Verification items for the finished model (mm, model axes). Face numbers are marked on the shaded views. A direction names the side the tool comes from. Give positions to 0.01 mm unless a question says otherwise; leave off trailing zeros. Write each loop counter-clockwise with the first axis right and the second up, starting at its lowest first coordinate (ties: lowest second). Pieces come first, ordered by that corner, then holes. Notation, with made-up numbers: (27, -16) -> (82, -16) arc R28 cw to (82, 21) -> close; hole circle Ø2 at (5.5, -3.75). An arc over 180 degrees is marked (long way). Answer as CSV lines item,"result".
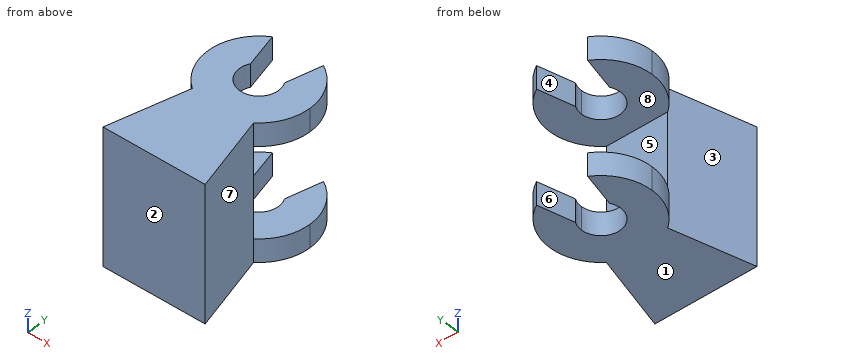
```python
from build123d import *

# Parameters (mm, degrees)
F1_DEPTH = 20
F2_DEPTH = 16.625
F3_DEPTH = 3.375


with BuildPart() as f1:
    # F0 (on Top) → F1 (new body)
    with BuildSketch(Plane.XY):
        with BuildLine():
            ThreePointArc((-11.25185, 21.143954), (-13.995725, 18.398907), (-15, 14.649832))
            ThreePointArc((-15, 14.649832), (-14.208204, 11.29573), (-12, 8.649832))
            Line((-12, 8.649832), (-3, 8.649832))
            ThreePointArc((-3, 8.649832), (-0.791796, 11.29573), (0, 14.649832))
            ThreePointArc((0, 14.649832), (-1.004275, 18.398907), (-3.74815, 21.143954))
            Line((-3.74815, 21.143954), (-5, 16.069559))
            ThreePointArc((-5, 16.069559), (-4.720331, 15.384041), (-4.625, 14.649832))
            ThreePointArc((-4.625, 14.649832), (-8.234209, 11.870163), (-10, 16.069559))
            Line((-10, 16.069559), (-11.25185, 21.143954))
        make_face()
        with BuildLine():
            Line((-12, 8.649832), (-15, -2.850168))
            Line((-15, -2.850168), (0, -2.850168))
            Line((0, -2.850168), (-3, 8.649832))
            ThreePointArc((-3, 8.649832), (-7.5, 7.149832), (-12, 8.649832))
        make_face()
        with BuildLine():
            Line((-3, 8.649832), (-12, 8.649832))
            ThreePointArc((-12, 8.649832), (-7.5, 7.149832), (-3, 8.649832))
        make_face()
    extrude(amount=F1_DEPTH)

    # F0 (on Top) → F2 (cut)
    with BuildSketch(Plane.XY):
        with BuildLine():
            ThreePointArc((-11.25185, 21.143954), (-13.995725, 18.398907), (-15, 14.649832))
            ThreePointArc((-15, 14.649832), (-14.208204, 11.29573), (-12, 8.649832))
            Line((-12, 8.649832), (-3, 8.649832))
            ThreePointArc((-3, 8.649832), (-0.791796, 11.29573), (0, 14.649832))
            ThreePointArc((0, 14.649832), (-1.004275, 18.398907), (-3.74815, 21.143954))
            Line((-3.74815, 21.143954), (-5, 16.069559))
            ThreePointArc((-5, 16.069559), (-4.720331, 15.384041), (-4.625, 14.649832))
            ThreePointArc((-4.625, 14.649832), (-8.234209, 11.870163), (-10, 16.069559))
            Line((-10, 16.069559), (-11.25185, 21.143954))
        make_face()
    extrude(amount=F2_DEPTH, mode=Mode.SUBTRACT)

    # F0 (on Top) → F3 (join)
    with BuildSketch(Plane.XY):
        with BuildLine():
            ThreePointArc((-11.25185, 21.143954), (-13.995725, 18.398907), (-15, 14.649832))
            ThreePointArc((-15, 14.649832), (-14.208204, 11.29573), (-12, 8.649832))
            Line((-12, 8.649832), (-3, 8.649832))
            ThreePointArc((-3, 8.649832), (-0.791796, 11.29573), (0, 14.649832))
            ThreePointArc((0, 14.649832), (-1.004275, 18.398907), (-3.74815, 21.143954))
            Line((-3.74815, 21.143954), (-5, 16.069559))
            ThreePointArc((-5, 16.069559), (-4.720331, 15.384041), (-4.625, 14.649832))
            ThreePointArc((-4.625, 14.649832), (-8.234209, 11.870163), (-10, 16.069559))
            Line((-10, 16.069559), (-11.25185, 21.143954))
        make_face()
    extrude(amount=F3_DEPTH)


solid = f1.part
```
1) Draft check along Y on the marked faces 6, 7 and 8. Enter one of: +Y half, -Y half, draft (parallel to the pull), parting line (faces both ways), or undercut.
Reported:
face 6,"+Y half"
face 7,"undercut"
face 8,"draft"
2) Section check D-D (z = 2). Record the boundary of the cut face in (x, y) (3 decimals), and give its area (3 significant figures).
Reported:
outline,"(-15, -2.85) -> (0, -2.85) -> (-3, 8.65) arc R7.5 ccw to (0, 14.65) arc R7.5 ccw to (-3.748, 21.144) -> (-5, 16.07) arc R2.875 cw to (-4.625, 14.65) arc R2.875 cw (long way) to (-10, 16.07) -> (-11.252, 21.144) arc R7.5 ccw to (-15, 14.65) arc R7.5 ccw to (-12, 8.65) -> close"
area,"248 mm²"
3) Scan lines: line 1 along Z through (x, y) = (-3, 18.25) (3 decimals); line 2 along Y through (x, z) = (-9.5, 9.75); line 3 along Y through (x, z) = (-7.5, 2.5). Record each from-to range of solid material in increasing order.
Reported:
line 1,"0 to 3.375, 16.625 to 20"
line 2,"-2.85 to 8.65"
line 3,"-2.85 to 11.77"
4) Depth check by flat-ended pin: pin 1 (4 mm diameter, centred on y = 8.5, z = 8.5, fed in from +X); pin 2 (1 mm diameter, centred on y = 6, z = 3.5, fed in from +X); pin 3 (4.5 mm diameter, centred on x = -9.5, z = 9, fed in from +Y). Enter the tip coordinate at first touch or a pass-through.
Reported:
pin 1,"x = -2.44"
pin 2,"x = -2.18"
pin 3,"y = 8.65"
5) Tool access check on the marked faces 1, 2, 3, 4 and 5. Record the directions out of +Z, -Z, +X, -X, +Y, -Y that give a thin tool (end or side, any length) a straight path to the whole face; none if there is none.
Reported:
face 1,"-Z, +X, -X, +Y, -Y"
face 2,"+Z, -Z, +X, -X, -Y"
face 3,"+Z, -Z, -X"
face 4,"+Z, -Z, +Y"
face 5,"+X, -X, +Y"
6) Section check C-C (y = 13). Record the boundary of the cut face in (x, z) (1 decimal).
Reported:
outline,"(-14.8, 0) -> (-9.9, 0) -> (-9.9, 3.4) -> (-14.8, 3.4) -> close; (-14.8, 16.6) -> (-9.9, 16.6) -> (-9.9, 20) -> (-14.8, 20) -> close; (-5.1, 0) -> (-0.2, 0) -> (-0.2, 3.4) -> (-5.1, 3.4) -> close; (-5.1, 16.6) -> (-0.2, 16.6) -> (-0.2, 20) -> (-5.1, 20) -> close"
7) Section check A-A (y = 10). Record the boundary of the cut face in (x, z) (3 decimals), and give its area (3 significant figures).
Reported:
outline,"(-13.385, 0) -> (-1.615, 0) -> (-1.615, 3.375) -> (-13.385, 3.375) -> close; (-13.385, 16.625) -> (-1.615, 16.625) -> (-1.615, 20) -> (-13.385, 20) -> close"
area,"79.4 mm²"
8) Section check B-B (x = -2.5). Record the boundary of the cut face in (y, z) (3 decimals), and give its area (3 significant figures).
Reported:
outline,"(-2.85, 0) -> (6.733, 0) -> (6.733, 20) -> (-2.85, 20) -> close; (9.06, 0) -> (20.24, 0) -> (20.24, 3.375) -> (9.06, 3.375) -> close; (9.06, 16.625) -> (20.24, 16.625) -> (20.24, 20) -> (9.06, 20) -> close"
area,"267 mm²"
